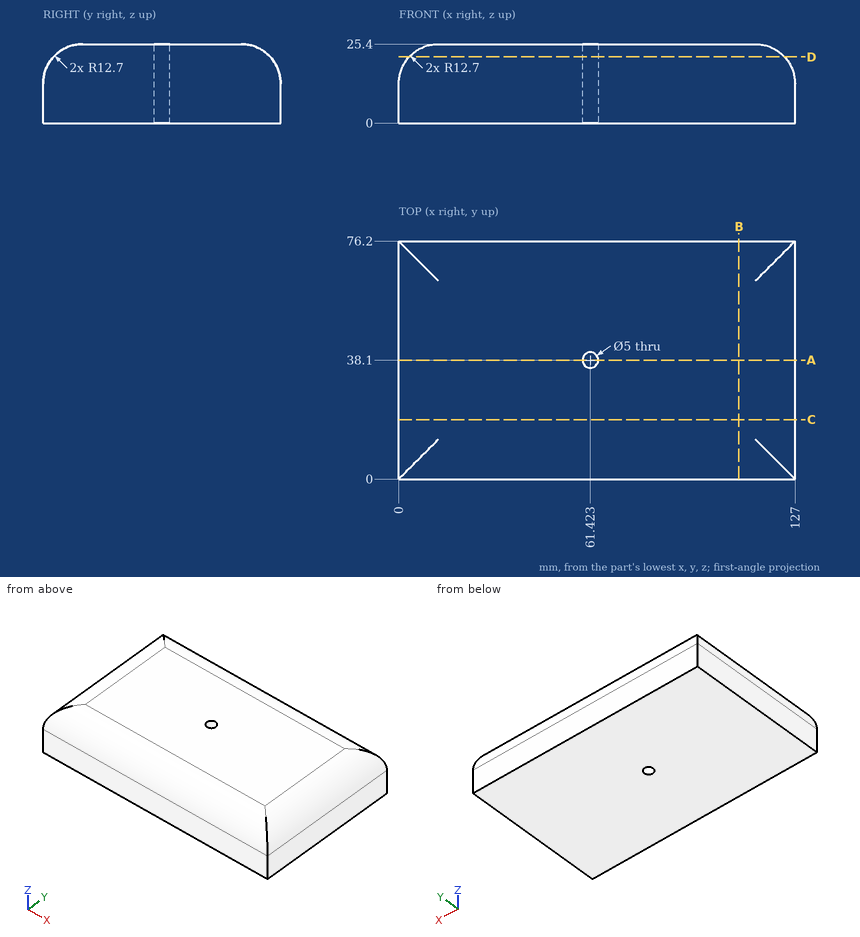
Drawing for the job (mm, zero at the part's lowest x, y, z). Round coordinates to 2 decimals unless told otherwise and drop trailing zeros. Write each loop counter-clockwise with the first axis right and the second up, starting at its lowest first coordinate (ties: lowest second). Pieces come first, ordered by that corner, then holes. Notation, with made-up numbers: M -29.75,67 L 26.25,67 A31 cw 26.25,91 Z; hole C 37.5,12 d3. An arc over 180 degrees is marked long. Answer in a Markdown table with one row per item.
1. Saw through at C-C (y = 19). List the corners of the cut face in (x, z), and give its area (3 significant figures).
Geometry check:
| item | result |
|---|---|
| outline | M 0,0 L 127,0 L 127,12.7 A12.7 ccw 114.3,25.4 L 12.7,25.4 A12.7 ccw 0,12.7 Z |
| area | 3,160 mm2 |
2. Saw through at B-B (x = 109). List the corners of the cut face in (y, z), and give its area (3 significant figures).
Geometry check:
| item | result |
|---|---|
| outline | M 0,0 L 76.2,0 L 76.2,12.7 A12.7 ccw 63.5,25.4 L 12.7,25.4 A12.7 ccw 0,12.7 Z |
| area | 1,870 mm2 |
3. Probe L1, parallel to Y at x = 68.5, z = 16; L2, parallel to Z at x = 56, y = 71.5; L3, parallel to Z at x = 34.5, y = 11. List the from-to ranges inside material, lowest first. Write a range as [from, to].
Geometry check:
| item | result |
|---|---|
| L1 | [0.44, 75.76] |
| L2 | [0, 22.56] |
| L3 | [0, 25.29] |
4. Flat gauge pins, fed straight in: P1, Ø4, axis at x = 23.5, y = 13.5, coming from the -Z side; P2, Ø3, axis at x = 61.42, y = 38.1, coming from the +Z side; P3, Ø1.5, axis at x = 73.5, z = 19.5, coming from the -Y side. Where does each tip first touch, or does it go through?
Geometry check:
| item | result |
|---|---|
| P1 | z = 0 |
| P2 | through |
| P3 | y = 1.53 |
5. Saw through at A-A (y = 38.1). List the corners of the cut face in (x, z).
Geometry check:
| item | result |
|---|---|
| outline | M 0,0 L 58.92,0 L 58.92,25.4 L 12.7,25.4 A12.7 ccw 0,12.7 Z; M 63.92,0 L 127,0 L 127,12.7 A12.7 ccw 114.3,25.4 L 63.92,25.4 Z |
6. Saw through at D-D (z = 21.25). List the corners of the cut face in (x, y).
Geometry check:
| item | result |
|---|---|
| outline | M 3.31,3.31 L 123.69,3.31 L 123.69,72.89 L 3.31,72.89 Z; hole C 61.42,38.1 d5 |
